For this review, take the finished solid that the model builds, in its own axes (mm). A direction names the side the tool comes from. Round coordinates to 2 decimals unless told otherwise and drop trailing zeros. Loops run counter-clockwise (first coordinate to the right, second up) from the corner with the lowest first, then second, coordinate; pieces in that order, holes last.
1) Take a section at B-B (y = -0.5). State the section outline as (x, z) points.
2) Take a section at A-A (x = 7). State the section outline as (y, z) points, then the cut area to 3 significant figures.
3) Take a section at D-D (y = 29). State the section outline as (x, z) points, then the cut area to 3 significant figures.
4) Mouldability with a two-part tool opening along X and no side actions: class faces 6 (the flat face through (27.75, 32, -7)), 7 (the flat face through (-38.14, -31.39, 1.48)), 8 (the flat face through (-1, 24, 5)) as pulls with the +X half, pulls with the -X half, needs draft (parallel to the pull), parting line crosses it, or undercut.
5) Tool access review of faces 1 (the flat face through (30.5, 0, 2)), 2 (the flat face through (-27.75, 32, -7)), 3 (the flat face through (-38.9, -31.1, 3)), 4 (the flat face through (-23, 30, -7)), 5 (the flat face through (-21.356, -31.479, -2.63)): name each direction out of +Z, -Z, +X, -X, +Y, -Y from which nothing blocks a thin tool from reaching the whole face with its end or side.
6) Take a section at C-C (z = -10.75). State the section outline as (x, y) points, then the cut area to 3 significant figures.
7) Wall thickness on L1, parallel to X at y = 29.5, z = 2.25; L2, parallel to Y at x = 39.5, z = 4.55; L3, parallel to Y at x = 3, z = 2.5: over which ranges is each line inside the solid? List them lowest first.
8) Insertion check: pin 1 (1.2 mm diameter, centred on x = 33.5, y = -22.5, fed in from +Z); pin 2 (0.9 mm diameter, centred on y = -32, z = -5, fed in from +X); pin 3 (4 mm diameter, centred on x = 2.5, z = -0.5, fed in from -Y); pin 4 (4 mm diameter, centred on y = 32.5, z = -6, fed in from -X). Each pin has a flat end and moves straight along its axis. Give the tip position at first contact, or say it passes through.
Autodesk Inventor part; units mm, degrees
ref_plane "YZ Plane" through (0, 0, 0) normal (1, 0, 0) x (0, 1, 0)
ref_plane "XZ Plane" through (0, 0, 0) normal (0, 1, 0) x (-1, 0, 0)
ref_plane "XY Plane" through (0, 0, 0) normal (0, 0, 1) x (1, 0, 0)
sketch "Sketch1" plane through (0, 0, 0) normal (0, 0, 1) x (1, 0, 0)
  line L0 (-30.5, -20) -> (30.5, -20)
  line L1 (30.5, -20) -> (30.5, 20)
  line L2 (30.5, 20) -> (-30.5, 20)
  line L3 (-30.5, 20) -> (-30.5, -20)
  line L4 (-30.5, -20) -> (30.5, 20) construction
  line L5 (30.5, -20) -> (-30.5, 20) construction
  line L6 (-45.5, -35) -> (45.5, -35)
  line L7 (45.5, -35) -> (45.5, 35)
  line L8 (45.5, 35) -> (-45.5, 35)
  line L9 (-45.5, 35) -> (-45.5, -35)
  line L10 (-45.5, -35) -> (45.5, 35) construction
  line L11 (45.5, -35) -> (-45.5, 35) construction
  point P0 (0, 0)
  dimension "d0" = 61
  dimension "d1" = 40
  dimension "d2" = 15
  dimension "d3" = 15
extrude "Rim" add sketch "Sketch1" along normal blind 5
sketch "Sketch2" plane through (0, 0, 5) normal (0, 0, 1) x (1, 0, 0)
  line L0 (-33.7, -22.765) -> (33.7, -22.765) construction
  line L1 (33.7, -22.765) -> (33.7, 22.765) construction
  line L2 (33.7, 22.765) -> (-33.7, 22.765) construction
  line L3 (-33.7, 22.765) -> (-33.7, -22.765) construction
  line L4 (-33.7, -22.765) -> (33.7, 22.765) construction
  line L5 (33.7, -22.765) -> (-33.7, 22.765) construction
  circle A0 centre (33.7, 22.765) radius 1.25
  line L6 (0, 22.765) -> (0, -22.765) construction
  line L7 (-30.5, -20) -> (-30.5, 20)
  line L8 (-30.5, 0) -> (33.7, 0) construction
  circle A1 centre (-33.7, 22.765) radius 1.25
  circle A2 centre (33.7, -22.765) radius 1.25
  circle A3 centre (-33.7, -22.765) radius 1.25
  point P0 (0, 0)
  dimension "d6" = 67.4
  dimension "d7" = 45.53
  dimension "d8" = 2.5
extrude "Pegs" cut sketch "Sketch2" against normal blind 3
sketch "Sketch3" plane through (0, 0, 0) normal (0, 0, -1) x (-1, 0, 0)
  line L0 (-39.5, 25.8246) -> (-42.25, 27.4123)
  line L1 (-36.75, 27.4123) -> (-39.5, 25.8246)
  line L2 (-42.25, 27.4123) -> (-42.25, 30.5877)
  line L3 (-36.75, 30.5877) -> (-36.75, 27.4123)
  circle A0 centre (-39.5, 29) radius 2
  line L4 (-39.5, 32.1754) -> (-36.75, 30.5877)
  line L5 (-42.25, 30.5877) -> (-39.5, 32.1754)
  line L6 (-45.5, 35) -> (35.9035, 35)
  line L7 (-45.5, 35) -> (-45.5, 29)
  line L8 (-45.5, -35) -> (-45.5, 35)
  line L9 (-45.5, 29) -> (-39.5, 29) construction
  line L10 (-45.5, -35) -> (-45.5, 35)
  line L11 (-45.5, 35) -> (45.5, 35)
  line L12 (0, 35) -> (0, -35) construction
  line L13 (45.5, -35) -> (-45.5, -35)
  line L14 (-45.5, 0) -> (45.5, 0) construction
  line L15 (45.5, 35) -> (45.5, -35)
  line L16 (39.5, 25.8246) -> (42.25, 27.4123)
  line L17 (36.75, 27.4123) -> (39.5, 25.8246)
  line L18 (42.25, 27.4123) -> (42.25, 30.5877)
  line L19 (36.75, 30.5877) -> (36.75, 27.4123)
  circle A1 centre (39.5, 29) radius 2
  line L20 (39.5, 32.1754) -> (36.75, 30.5877)
  line L21 (42.25, 30.5877) -> (39.5, 32.1754)
  line L22 (45.5, 29) -> (39.5, 29) construction
  line L23 (-39.5, -25.8246) -> (-42.25, -27.4123)
  line L24 (-36.75, -27.4123) -> (-39.5, -25.8246)
  line L25 (-42.25, -27.4123) -> (-42.25, -30.5877)
  line L26 (-36.75, -30.5877) -> (-36.75, -27.4123)
  circle A2 centre (-39.5, -29) radius 2
  line L27 (-39.5, -32.1754) -> (-36.75, -30.5877)
  line L28 (-42.25, -30.5877) -> (-39.5, -32.1754)
  line L29 (36.75, -30.5877) -> (36.75, -27.4123)
  line L30 (39.5, -32.1754) -> (36.75, -30.5877)
  circle A3 centre (39.5, -29) radius 2
  line L31 (42.25, -30.5877) -> (39.5, -32.1754)
  line L32 (42.25, -27.4123) -> (42.25, -30.5877)
  line L33 (39.5, -25.8246) -> (42.25, -27.4123)
  line L34 (36.75, -27.4123) -> (39.5, -25.8246)
  point P0 (0, 0)
  dimension "d11" = 3.1754
  dimension "d12" = 4
  dimension "d13" = 6
  dimension "d14" = 6
extrude "Nut Hexes" cut sketch "Sketch3" against normal blind 3 contours L0 L2 L5 L4 L3 L1 | L17 L19 L20 L21 L18 L16 | L24 L26 L27 L28 L25 L23 | L29 L34 L33 L32 L31 L30
sketch "Sketch4" plane through (0, 0, 0) normal (0, 0, -1) x (-1, 0, 0)
  circle A0 centre (-39.5, 29) radius 2
  circle A1 centre (39.5, 29) radius 2
  circle A2 centre (39.5, -29) radius 2
  circle A3 centre (-39.5, -29) radius 2
  point P0 (0, 0)
extrude "Bolt Holes" cut sketch "Sketch4" against normal up to next
sketch "For Construction" plane through (0, 0, 5) normal (0, 0, 1) x (1, 0, 0)
  circle A0 centre (33.7, -22.765) radius 1.25
  circle A1 centre (39.5, -29) radius 2
  point P0 (0, 0)
  point P1 (34.95, -22.765)
  point P2 (37.901, -27.7986)
  dimension "d19" = 5.2656
sketch "Sketch7" plane through (0, 0, 0) normal (0, 0, -1) x (-1, 0, 0)
  line L0 (45.5, -35) -> (-45.5, -35)
  line L1 (45.5, -35) -> (0, -35)
  line L2 (27.75, -35) -> (17.75, -35)
  line L3 (17.75, -35) -> (17.75, -30)
  line L4 (17.75, -30) -> (27.75, -30)
  line L5 (27.75, -30) -> (27.75, -35)
  line L6 (0, -35) -> (0, 35.2559) construction
  line L7 (-27.75, -35) -> (-17.75, -35)
  line L8 (-17.75, -35) -> (-17.75, -30)
  line L9 (-17.75, -30) -> (-27.75, -30)
  line L10 (-27.75, -30) -> (-27.75, -35)
  point P0 (0, 0)
  point P1 (22.75, -35)
  point P2 (-22.75, -35)
  dimension "d20" = 5
  dimension "d21" = 10
extrude "Attachment Points" add sketch "Sketch7" along normal blind 10
sketch "Sketch9" plane through (-45.5, -35, 5) normal (0, -1, 0) x (1, 0, 0)
  circle A0 centre (22.75, -10) radius 2
  circle A1 centre (68.25, -10) radius 2
  point P0 (45.5, -5)
  point P1 (22.75, -8)
  point P2 (68.25, -8)
extrude "Connection Holes" cut sketch "Sketch9" against normal up to next
sketch "Sketch10" plane through (0, 0, 0) normal (0, 0, -1) x (-1, 0, 0)
  line L0 (45.5, 35) -> (45.5, -35)
  line L1 (-45.5, -35) -> (-45.5, 35)
  line L2 (-45.5, 35) -> (45.5, 35)
  line L3 (0, 35) -> (45.5, 35)
  line L4 (0, 35) -> (-45.5, 35)
  line L5 (45.5, -5) -> (40.5, -5)
  line L6 (40.5, -5) -> (40.5, 5)
  line L7 (40.5, 5) -> (45.5, 5)
  line L8 (45.5, 5) -> (45.5, -5)
  line L9 (17.75, -35) -> (-17.75, -35)
  line L10 (0, -35) -> (0, -19.876) construction
  line L11 (-45.5, 35) -> (-45.5, -35)
  line L12 (-45.5, -5) -> (-40.5, -5)
  line L13 (-40.5, -5) -> (-40.5, 5)
  line L14 (-40.5, 5) -> (-45.5, 5)
  line L15 (-45.5, 5) -> (-45.5, -5)
  line L16 (27.75, 35) -> (17.75, 35)
  line L17 (17.75, 35) -> (17.75, 30)
  line L18 (17.75, 30) -> (27.75, 30)
  line L19 (27.75, 30) -> (27.75, 35)
  line L20 (-27.75, 35) -> (-17.75, 35)
  line L21 (-17.75, 35) -> (-17.75, 30)
  line L22 (-17.75, 30) -> (-27.75, 30)
  line L23 (-27.75, 30) -> (-27.75, 35)
  point P0 (0, 0)
  point P1 (45.5, 0)
  point P2 (-45.5, 0)
  point P3 (22.75, 35)
  point P4 (-22.75, 35)
  point P5 (45.5, 0)
  point P6 (-45.5, 0)
  point P7 (-45.5, 0)
  dimension "d28" = 5
  dimension "d29" = 10
  dimension "d30" = 5
  dimension "d31" = 10
extrude "Legs 1" add sketch "Sketch10" along normal blind 15
sketch "Sketch11" plane through (0, 0, -10) normal (0, 0, -1) x (-1, 0, 0)
  line L0 (27.75, -30) -> (27.75, -35)
  line L1 (27.75, -30) -> (17.75, -30)
  line L2 (27.75, -35) -> (17.75, -35)
  line L3 (17.75, -35) -> (17.75, -30)
  line L4 (17.75, -30) -> (27.75, -30)
  line L5 (27.75, -30) -> (27.75, -35)
  line L6 (-17.75, -35) -> (-17.75, -30)
  line L7 (-27.75, -30) -> (-27.75, -35)
  line L8 (-17.75, -35) -> (-27.75, -35)
  line L9 (-27.75, -35) -> (-27.75, -30)
  line L10 (-27.75, -30) -> (-17.75, -30)
  line L11 (-17.75, -30) -> (-17.75, -35)
  point P0 (0, 0)
extrude "Extrusion9" add sketch "Sketch11" along normal blind 5
ref_plane "Work Plane2" through (-30.5, 0, 0) normal (0, 1, 0) x (1, 0, 0)
sketch "Sketch12" plane through (17.75, -30, 0) normal (0, 1, 0) x (1, 0, 0)
  line L0 (5, 1.8246) -> (2.25, 3.4123)
  line L1 (7.75, 3.4123) -> (5, 1.8246)
  line L2 (2.25, 3.4123) -> (2.25, 6.5877)
  line L3 (7.75, 6.5877) -> (7.75, 3.4123)
  line L4 (5, 8.1754) -> (7.75, 6.5877)
  line L5 (2.25, 6.5877) -> (5, 8.1754)
  circle A0 centre (5, 5) radius 2
  line L6 (0, 0) -> (0, 15)
  line L7 (-40.5, 1.8246) -> (-43.25, 3.4123)
  line L8 (-37.75, 3.4123) -> (-40.5, 1.8246)
  line L9 (-43.25, 3.4123) -> (-43.25, 6.5877)
  line L10 (-37.75, 6.5877) -> (-37.75, 3.4123)
  line L11 (-40.5, 8.1754) -> (-37.75, 6.5877)
  line L12 (-43.25, 6.5877) -> (-40.5, 8.1754)
  circle A1 centre (-40.5, 5) radius 2
  line L13 (-35.5, 0) -> (-35.5, 15)
  point P0 (-17.75, 0)
  point P1 (-5.2731, 15.8695)
  point P2 (-26.4318, 33.2663)
  dimension "d36" = 3.1754
  dimension "d38" = 3.1754
extrude "Extrusion10" cut sketch "Sketch12" against normal blind 3
properties part number "Joystickboard Holder"
Response:
1. outline: (-45.5, -15) - (-40.5, -15) - (-40.5, 0) - (-30.5, 0) - (-30.5, 5) - (-45.5, 5) - close; (30.5, 0) - (40.5, 0) - (40.5, -15) - (45.5, -15) - (45.5, 5) - (30.5, 5) - close
2. outline: (-35, 0) - (-20, 0) - (-20, 5) - (-35, 5) - close; (20, 0) - (35, 0) - (35, 5) - (20, 5) - close
2. area: 150 mm2
3. outline: (-45.5, 0) - (-42.25, 0) - (-42.25, 3) - (-41.5, 3) - (-41.5, 5) - (-45.5, 5) - close; (-37.5, 3) - (-36.75, 3) - (-36.75, 0) - (36.75, 0) - (36.75, 3) - (37.5, 3) - (37.5, 5) - (-37.5, 5) - close; (41.5, 3) - (42.25, 3) - (42.25, 0) - (45.5, 0) - (45.5, 5) - (41.5, 5) - close
3. area: 406 mm2
4. face 6: pulls with the +X half
4. face 7: undercut
4. face 8: needs draft
5. face 1: +Z, -Z
5. face 2: -Z, -X, +Y, -Y
5. face 3: -Z
5. face 4: -Z, +X, -X
5. face 5: none
6. outline: (-45.5, -5) - (-40.5, -5) - (-40.5, 5) - (-45.5, 5) - close; (-27.75, -35) - (-17.75, -35) - (-17.75, -30) - (-27.75, -30) - close; (-27.75, 30) - (-17.75, 30) - (-17.75, 35) - (-27.75, 35) - close; (17.75, -35) - (27.75, -35) - (27.75, -30) - (17.75, -30) - close; (17.75, 30) - (27.75, 30) - (27.75, 35) - (17.75, 35) - close; (40.5, -5) - (45.5, -5) - (45.5, 5) - (40.5, 5) - close
6. area: 300 mm2
7. L1: x = -45.5 to -42.25, -36.75 to 36.75, 42.25 to 45.5
7. L2: y = -35 to -31, -27 to 27, 31 to 35
7. L3: y = -35 to -20, 20 to 35
8. pin 1: stops at z = 2
8. pin 2: stops at x = 27.75
8. pin 3: stops at y = -35
8. pin 4: stops at x = -27.75
